Answer from the drawing. Dimensions are ordinates in mm from the lowest x, y and z of the part. Round coordinates to 2 decimals unless told otherwise and drop trailing zeros. Loops run counter-clockwise (first coordinate to the right, second up) from the corner with the lowest first, then second, coordinate; pieces in that order, holes last.
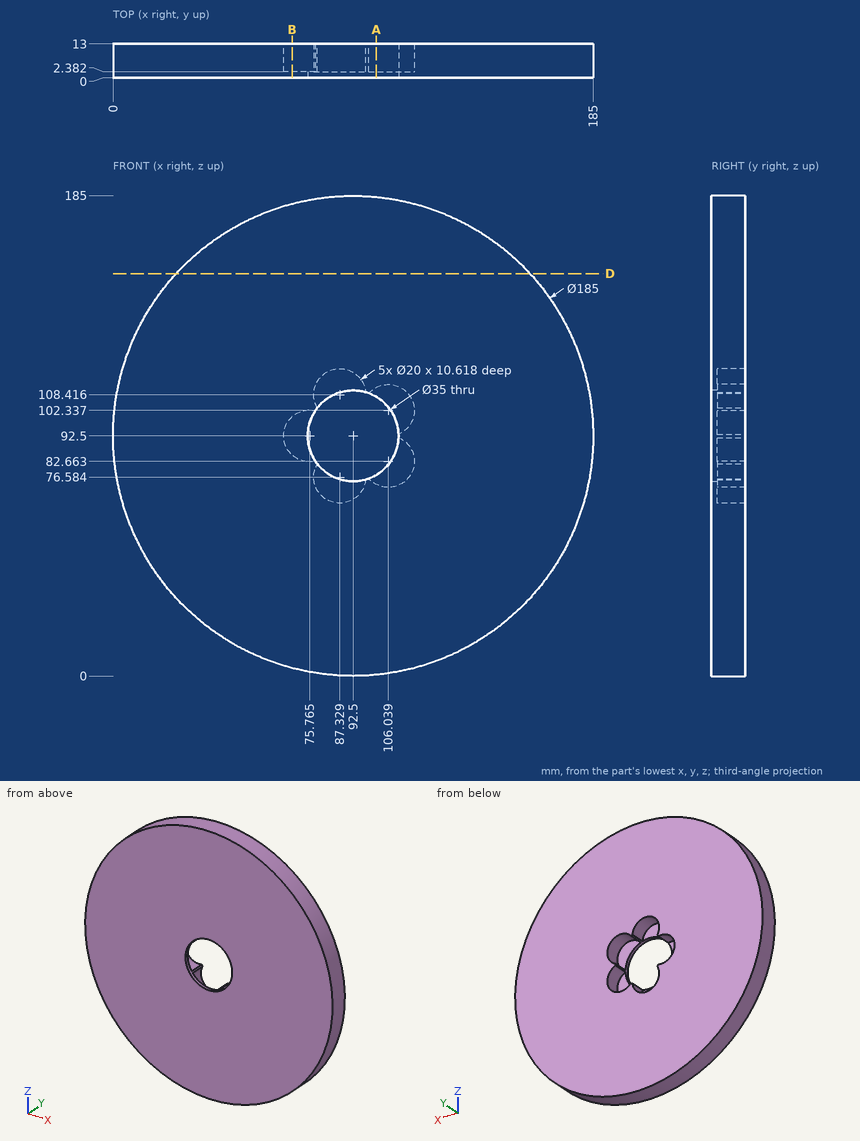
1. Find section B-B (x = 69). Write down the section's boundary in (y, z) (1 decimal), then the cut area to 3 significant figures.
Answer key:
outline: (0, 3) - (13, 3) - (13, 85.1) - (2.4, 85.1) - (2.4, 99.9) - (13, 99.9) - (13, 182) - (0, 182) - close
area: 2,170 mm2
2. Given pin 1 (1.5 mm diameter, centred on y = 8, z = 150.5, fed in from -X) (1 decimal); pin 2 (5 mm diameter, centred on y = 10, z = 116, fed in from -X) (1 decimal); pin 3 (12 mm diameter, centred on x = 86, z = 111.5, fed in from +Y), each flat-ended and moving along its own axis, determine where each tip first touches the part or whether it passes through.
Answer key:
pin 1: stops at x = 19.8
pin 2: stops at x = 2.4
pin 3: stops at y = 2.38
3. Find section D-D (z = 155). Write down the section's boundary in (x, y).
Answer key:
outline: (24.31, 0) - (160.69, 0) - (160.69, 13) - (24.31, 13) - close
4. Find section A-A (x = 101.5). Write down the section's boundary in (y, z).
Answer key:
outline: (0, 0.44) - (13, 0.44) - (13, 73.75) - (2.38, 73.75) - (2.38, 77.49) - (0, 77.49) - close; (0, 107.51) - (2.38, 107.51) - (2.38, 111.25) - (13, 111.25) - (13, 184.56) - (0, 184.56) - close
5. Consider probe 1 along X at (y, z) = (4, 92.5) (1 decimal); probe 2 along Z at (x, y) = (73, 9.75); probe 3 along Z at (x, y) = (72.5, 7). Determine where each line is inside the solid, lowest interval first.
Answer key:
probe 1: x = 0 to 65.8, 110 to 185
probe 2: z = 2.08 to 82.89, 102.11 to 182.92
probe 3: z = 2.19 to 83.05, 101.95 to 182.81
